Verification items for the finished model (mm, model axes). Coordinates: 2 decimals unless noted, no trailing zeros. Write each loop counter-clockwise with the first axis right and the second up, starting at its lowest first coordinate (ties: lowest second). Pieces come first, ordered by that corner, then holes. Notation, with made-up numbers: (-21, 61.25) -> (13, 61.25) arc R20 cw to (13, 85.25) -> close; hole circle Ø2 at (-1.75, -29). An arc over 180 degrees is marked (long way). Use a Markdown table: item, result. Add a question column.
from build123d import *

# Parameters (mm, degrees)
F1_DEPTH = 15
F3_D     = 20.5


with BuildPart() as f1:
    # F0 (on Top) → F1 (new body)
    with BuildSketch(Plane.XY):
        Polygon((72.9636595731, 490.75858604), (0, 0), (125, 0), (125, 490.75858604), align=None)
        Polygon((125, 490.75858604), (125, 0), (250, 0), (177.0363404269, 490.75858604), align=None)
    extrude(amount=F1_DEPTH)

    # F3 (through all)
    with Locations(Plane(origin=(0, 0, 0), x_dir=(1, 0, 0), z_dir=(0, 0, -1))):
        with Locations((125, -450), (62, -243), (188, -243), (191, -40), (59, -40)):
            Hole(F3_D / 2)


solid = f1.part
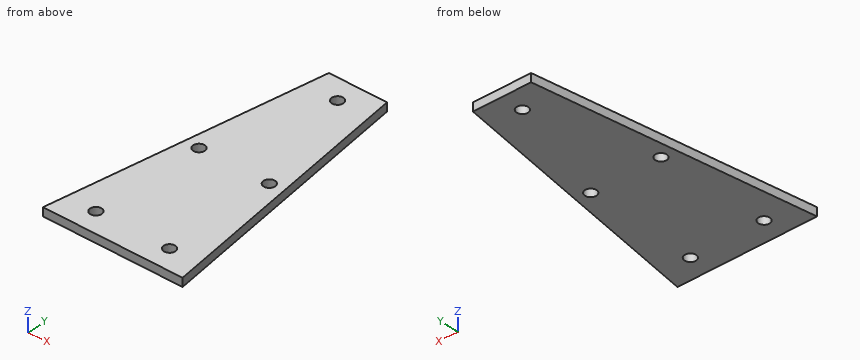
1) Cross-section at C-C on y = 450. Record the boundary of the cut face in (x, z), then the cut area to 3 significant figures.
2) Gauge pin test, flat ends, axial feed: pin 1 (3 mm diameter, centred on y = 262, z = 12.5, fed in from -X); pin 2 (4 mm diameter, centred on y = 338, z = 10.5, fed in from -X); pin 3 (12.5 mm diameter, centred on x = 188, y = 243, fed in from +Z); pin 4 (4 mm diameter, centred on y = 284, z = 10, fed in from -X). Record the tip position at first contact, or that the pin passes through.
3) Cross-section at A-A on z = 5.5. Record the boundary of the cut face in (x, y), then the cut area to 3 significant figures.
4) Thickness scan on L1, parallel to Y at x = 125, z = 3.25; L2, parallel to X at y = 40, z = 8; L3, parallel to Y at x = 134, z = 10. Record the ranges inside material, lowest first.
5) Cross-section at B-B on x = 188. Record the boundary of the cut face in (y, z), then the cut area to 3 significant figures.
6) Cross-section at D-D on x = 125. Record the boundary of the cut face in (y, z), then the cut area to 3 significant figures.
Returned:
| question | item | result |
|---|---|---|
| 1 | outline | (66.9, 0) -> (114.75, 0) -> (114.75, 15) -> (66.9, 15) -> close; (135.25, 0) -> (183.1, 0) -> (183.1, 15) -> (135.25, 15) -> close |
| 1 | area | 1,440 mm² |
| 2 | pin 1 | stops at x = 38.73 |
| 2 | pin 2 | stops at x = 49.95 |
| 2 | pin 3 | passes through |
| 2 | pin 4 | stops at x = 41.93 |
| 3 | outline | (0, 0) -> (250, 0) -> (177.04, 490.76) -> (72.96, 490.76) -> close; hole circle Ø20.5 at (59, 40); hole circle Ø20.5 at (62, 243); hole circle Ø20.5 at (125, 450); hole circle Ø20.5 at (188, 243); hole circle Ø20.5 at (191, 40) |
| 3 | area | 85,200 mm² |
| 4 | L1 | y = 0 to 439.75, 460.25 to 490.76 |
| 4 | L2 | x = 5.95 to 48.75, 69.25 to 180.75, 201.25 to 244.05 |
| 4 | L3 | y = 0 to 445.09, 454.91 to 490.76 |
| 5 | outline | (0, 0) -> (30.2, 0) -> (30.2, 15) -> (0, 15) -> close; (49.8, 0) -> (232.75, 0) -> (232.75, 15) -> (49.8, 15) -> close; (253.25, 0) -> (417.02, 0) -> (417.02, 15) -> (253.25, 15) -> close |
| 5 | area | 5,650 mm² |
| 6 | outline | (0, 0) -> (439.75, 0) -> (439.75, 15) -> (0, 15) -> close; (460.25, 0) -> (490.76, 0) -> (490.76, 15) -> (460.25, 15) -> close |
| 6 | area | 7,050 mm² |
